```python
from build123d import *

# Parameters (mm, degrees)
SKETCH_1_R          = 27.5
EXTRUDE_1_DEPTH     = 1
SKETCH_2_R          = 25.25
EXTRUDE_2_DEPTH     = 7
SKETCH_3_R          = 27.5
EXTRUDE_3_DEPTH     = 1
SKETCH_4_R          = 17.5
EXTRUDE_4_DEPTH     = 7
SKETCH_5_R          = 4
CUT_EXTRUDE_1_DEPTH = 100
SKETCH_6_R          = 1.25
CUT_EXTRUDE_2_DEPTH = 100


with BuildPart() as part:
    # 草图1 → 凸台-拉伸1 (new body)
    with BuildSketch(Plane.XY):
        Circle(SKETCH_1_R)
    extrude(amount=EXTRUDE_1_DEPTH)

    # 草图2 → 凸台-拉伸2 (add)
    with BuildSketch(Plane.XY.offset(1)):
        Circle(SKETCH_2_R)
    extrude(amount=EXTRUDE_2_DEPTH)

    # 草图3 → 凸台-拉伸3 (add)
    with BuildSketch(Plane.XY.offset(8)):
        Circle(SKETCH_3_R)
    extrude(amount=EXTRUDE_3_DEPTH)

    # 草图4 → 凸台-拉伸4 (add)
    with BuildSketch(Plane.XY.offset(9)):
        Circle(SKETCH_4_R)
    extrude(amount=EXTRUDE_4_DEPTH)

    # 草图5 → 切除-拉伸1 (cut)
    with BuildSketch(Plane.XY.offset(16)):
        Circle(SKETCH_5_R)
    extrude(amount=-CUT_EXTRUDE_1_DEPTH, mode=Mode.SUBTRACT)

    # 草图6 → 切除-拉伸2 (cut)
    with BuildSketch(Plane(origin=(0, 0, 0), x_dir=(-1, 0, 0), z_dir=(0, 0, -1))):
        with Locations((7, 0)):
            Circle(SKETCH_6_R)
        with Locations((0, -7)):
            Circle(SKETCH_6_R)
        with Locations((-7, 0)):
            Circle(SKETCH_6_R)
        with Locations((0, 7)):
            Circle(SKETCH_6_R)
    extrude(amount=-CUT_EXTRUDE_2_DEPTH, mode=Mode.SUBTRACT)


solid = part.part
```
Work out the finished part from the listing and answer in its coordinate system (mm). A direction names the side the tool comes from. Round coordinates to 2 decimals unless told otherwise and drop trailing zeros. Write each loop counter-clockwise with the first axis right and the second up, starting at its lowest first coordinate (ties: lowest second). Pieces come first, ordered by that corner, then holes. Notation, with made-up numbers: (67, 83.25) -> (116, 83.25) arc R9 ccw to (116, 93.25) -> close; hole circle Ø6 at (-28, -11). An arc over 180 degrees is marked (long way). Write each question's results on one line, items separated by ' | '.
Q1. Which of the six approach directions +Z, -Z, +X, -X, +Y, -Y give full straight-line access (tool end or side, diameter ignored) to faces 1 (the flat face through (8, -24.3, 8)), 2 (the flat face through (0, -18, 9)), 3 (the cylindrical face through (0.27, -8.22, 7.89))?
Data:
face 1: none | face 2: +Z | face 3: +Z, -Z
Q2. Flat-ended cylindrical pins translate along their axes: P1, Ø6.5, axis at x = 0, y = 0, coming from the +Z side; P2, Ø1.5, axis at x = -12, y = 14, coming from the +Z side; P3, Ø2, axis at y = 14, z = 11, coming from the -X side; P4, Ø2, axis at y = -15, z = 10.5, coming from the -X side. Find the tip coordinate at first contact, or state that the pin passes through.
Data:
P1: through | P2: z = 9 | P3: x = -11.72 | P4: x = -10.5
Q3. Section D-D, the plane x = -6.5 is taken. Write down the section's boundary in (y, z).
Data:
outline: (-26.72, 0) -> (-1.15, 0) -> (-1.15, 16) -> (-16.25, 16) -> (-16.25, 9) -> (-26.72, 9) -> (-26.72, 8) -> (-24.4, 8) -> (-24.4, 1) -> (-26.72, 1) -> close; (1.15, 0) -> (26.72, 0) -> (26.72, 1) -> (24.4, 1) -> (24.4, 8) -> (26.72, 8) -> (26.72, 9) -> (16.25, 9) -> (16.25, 16) -> (1.15, 16) -> close
Q4. Straight lines are drawn through the part: line 1 along Y through (x, z) = (0, 8.5); line 2 along Y through (x, z) = (0, 3); line 3 along X through (y, z) = (-0.5, 3.75). For each, find the intervals that lie inside material, in ascending order. Write a range as [from, to].
Data:
line 1: [-27.5, -8.25], [-5.75, -4], [4, 5.75], [8.25, 27.5] | line 2: [-25.25, -8.25], [-5.75, -4], [4, 5.75], [8.25, 25.25] | line 3: [-25.25, -8.15], [-5.85, -3.97], [3.97, 5.85], [8.15, 25.25]
Q5. Determine the mould class of faces 4 (the cylindrical face through (-5.47, -24.65, 4.45)), 5 (the cylindrical face through (-0.867, -3.905, 8.112)), 6 (the flat face through (4, -4, 16)) for opening direction Z: released by +Z, released by -Z, zero draft, split by the parting line, or undercut.
Data:
face 4: undercut | face 5: zero draft | face 6: released by +Z
Q6. Section A-A, the plane x = 0 is taken. Write down the section's boundary in (y, z), then the cut area to 4 significant figures.
Data:
outline: (-27.5, 0) -> (-8.25, 0) -> (-8.25, 16) -> (-17.5, 16) -> (-17.5, 9) -> (-27.5, 9) -> (-27.5, 8) -> (-25.25, 8) -> (-25.25, 1) -> (-27.5, 1) -> close; (-5.75, 0) -> (-4, 0) -> (-4, 16) -> (-5.75, 16) -> close; (4, 0) -> (5.75, 0) -> (5.75, 16) -> (4, 16) -> close; (8.25, 0) -> (27.5, 0) -> (27.5, 1) -> (25.25, 1) -> (25.25, 8) -> (27.5, 8) -> (27.5, 9) -> (17.5, 9) -> (17.5, 16) -> (8.25, 16) -> close | area: 500.5 mm^2
Q7. Section C-C, the plane y = -7 is taken. Write down the section's boundary in (x, z), then the cut area to 3 significant figures.
Data:
outline: (-26.59, 0) -> (-1.25, 0) -> (-1.25, 16) -> (-16.04, 16) -> (-16.04, 9) -> (-26.59, 9) -> (-26.59, 8) -> (-24.26, 8) -> (-24.26, 1) -> (-26.59, 1) -> close; (1.25, 0) -> (26.59, 0) -> (26.59, 1) -> (24.26, 1) -> (24.26, 8) -> (26.59, 8) -> (26.59, 9) -> (16.04, 9) -> (16.04, 16) -> (1.25, 16) -> close | area: 631 mm^2
Q8. Section B-B, the plane z = 10.25 is taken. Write down the section's boundary in (x, y).
Data:
outline: circle Ø35 at (0, 0); hole circle Ø2.5 at (-7, 0); hole circle Ø8 at (0, 0); hole circle Ø2.5 at (0, -7); hole circle Ø2.5 at (0, 7); hole circle Ø2.5 at (7, 0)
